Autodesk Inventor part; units mm, degrees
ref_plane "YZ Plane" through (0, 0, 0) normal (1, 0, 0) x (0, 1, 0)
ref_plane "XZ Plane" through (0, 0, 0) normal (0, 1, 0) x (-1, 0, 0)
ref_plane "XY Plane" through (0, 0, 0) normal (0, 0, 1) x (1, 0, 0)
sketch "Skizze1" plane through (0, 0, 0) normal (0, 1, 0) x (-1, 0, 0)
  line L0 (-27, 70) -> (27, 70)
  line L1 (27, 70) -> (27, -70)
  line L2 (27, -70) -> (-27, -70)
  line L3 (-27, -70) -> (-27, 70)
  line L4 (-27, 70) -> (27, -70) construction
  line L5 (27, 70) -> (-27, -70) construction
  point P0 (0, 0)
  dimension "d0" = 54
  dimension "d1" = 140
extrude "Extrusion1" add sketch "Skizze1" along normal blind 15
sketch "Skizze2" plane through (0, 15, 0) normal (0, 1, 0) x (1, 0, 0)
  line L0 (24, -63) -> (-24, -63)
  line L1 (-24, -63) -> (-24, 63)
  line L2 (-24, 63) -> (24, 63)
  line L3 (24, 63) -> (24, -63)
  line L4 (24, -63) -> (-24, 63) construction
  line L5 (-24, -63) -> (24, 63) construction
  line L6 (-27, -70) -> (27, -70)
  line L7 (27, -70) -> (27, 70)
  line L8 (27, 70) -> (-27, 70)
  line L9 (-27, 70) -> (-27, -70)
  point P0 (0, 0)
  dimension "d4" = 3
  dimension "d7" = 7
extrude "Extrusion2" cut sketch "Skizze2" against normal blind 12 contours L0 L1 L2 L3
sketch "Skizze4" plane through (-27, 0, 70) normal (0, 0, 1) x (1, 0, 0)
  line L0 (54, 0) -> (0, 0)
  line L1 (54, 0) -> (54, 15)
  line L2 (0, 15) -> (54, 15)
  line L3 (0, 0) -> (0, 15)
  point P0 (27, 3.5)
  dimension "d23" = 3.5
hole "Bohrung1" at (0, 3.5, 70) direction (0, 0, -1) diameter 2.459 depth 5 tip angle 118
pattern_linear "Rechteckige Anordnung1" count 5 spacing 11 along (-1, 0, 0) count 2 spacing 8 along (0, 1, 0) of "Bohrung1" first direction both ways yes
mirror "Spiegeln1" about plane through (0, 0, 0) normal (0, 0, 1) of "Extrusion2", "Bohrung1", "Rechteckige Anordnung1"
sketch "Skizze6" plane through (0, 0, 0) normal (0, -1, 0) x (1, 0, 0)
  line L0 (-18, 18) -> (18, 18)
  line L1 (18, 18) -> (18, -18)
  line L2 (18, -18) -> (-18, -18)
  line L3 (-18, -18) -> (-18, 18)
  line L4 (-18, 18) -> (18, -18) construction
  line L5 (18, 18) -> (-18, -18) construction
  line L6 (0, 18) -> (0, -18) construction
  line L7 (-18, 0) -> (18, 0) construction
  point P0 (0, 0)
  dimension "d47" = 36
  dimension "d48" = 36
hole "Bohrung2" at (18, 0, 18) at (18, 0, 0) at (18, 0, -18) at (0, 0, -18) at (-18, 0, -18) at (-18, 0, 0) at (-18, 0, 18) at (0, 0, 18) direction (0, 1, 0) diameter 2.459 depth 8.8 tip angle 118
fillet "Rundung2" radius 4 4 edges at (-24, 9, -63) (24, 9, -63) (24, 9, 63) (-24, 9, 63)
properties part number "dynamixel_pro_frame_part1" material "Aluminium 6061"
Build history of the part. All positions in model axes, mm. A direction names the side the tool comes from. Coordinates: 2 decimals unless noted, no trailing zeros. Order: outer loops, then holes, each group sorted by start corner. A loop starts at its lowest first (then second) coordinate and runs counter-clockwise, first axis right, second up. Notation, with made-up numbers: (62.5, 23.25) -> (81.5, 23.25) arc R11 ccw to (81.5, 36.25) -> close; hole circle Ø8 at (28.25, -31). An arc over 180 degrees is marked (long way). Answer in a Markdown table with one row per item. Add a question column.
Q1. Mould opens along Z. For faces 6 (the face through (-22.797, 8.916, 61.859)), 7 (the face through (10.631, 10.327, 67.465)), 8 (the face through (11.18, 11.39, 64.39)) say: +Z half, -Z half, draft (parallel to the pull), parting line (faces both ways), or undercut.
Q2. Wall check: line 1 along X through (y, z) = (11.5, 67.2); line 2 along Y through (x, z) = (11, -66.4); line 3 along X through (y, z) = (1.65, 18). Give the ranges that are in metal, low to high. Write a range as [from, to].
Q3. Band-saw the part on B-B, the plane z = 32. List the corners of the cut face in (x, y).
Q4. Band-saw the part on C-C, the plane x = 2.5. List the corners of the cut face in (y, z).
Q5. Which spindle directions (+Z, -Z, +X, -X, +Y, -Y) get a long thin tool onto all of the face, cutting with end or side? Do faces 1 (the face through (0.05, 4.73, -67.46)), 2 (the face through (-27, 7, 1)), 3 (the face through (0, 9, 63)), 4 (the face through (23.2, 3.77, 67.46)), 5 (the face through (0.471, 1.521, -19.136)). Say none if no direction does.
Q6. Band-saw the part on A-A, the plane z = -18. List the corners of the cut face in (x, y), then the cut area to 3 significant figures.
Q7. Drop flat-ended pins along their axis: pin 1 (1.5 mm diameter, centred on x = 11, y = 11.5, fed in from -Z); pin 2 (1.5 mm diameter, centred on x = 11, y = 3.5, fed in from +Z); pin 3 (1.5 mm diameter, centred on x = 17.5, z = 16, fed in from +Y); pin 4 (2 mm diameter, centred on x = 0, z = -18, fed in from +Y). Give the stop position or say it passes through.
Answers follow:
| question | item | result |
|---|---|---|
| 1 | face 6 | undercut |
| 1 | face 7 | draft |
| 1 | face 8 | +Z half |
| 2 | line 1 | [-27, -23.23], [-20.77, -12.23], [-9.77, -1.23], [1.23, 9.77], [12.23, 20.77], [23.23, 27] |
| 2 | line 2 | [0, 2.27], [4.73, 10.27], [12.73, 15] |
| 2 | line 3 | [-27, -19.23], [-16.77, -1.23], [1.23, 16.77], [19.23, 27] |
| 3 | outline | (-27, 0) -> (27, 0) -> (27, 15) -> (24, 15) -> (24, 3) -> (-24, 3) -> (-24, 15) -> (-27, 15) -> close |
| 4 | outline | (0, -70) -> (15, -70) -> (15, -63) -> (3, -63) -> (3, 63) -> (15, 63) -> (15, 70) -> (0, 70) -> close |
| 5 | face 1 | -Z |
| 5 | face 2 | +Z, -Z, -X, +Y, -Y |
| 5 | face 3 | +Y |
| 5 | face 4 | +Z |
| 5 | face 5 | +Y, -Y |
| 6 | outline | (-27, 0) -> (-19.23, 0) -> (-19.23, 3) -> (-24, 3) -> (-24, 15) -> (-27, 15) -> close; (-16.77, 0) -> (-1.23, 0) -> (-1.23, 3) -> (-16.77, 3) -> close; (1.23, 0) -> (16.77, 0) -> (16.77, 3) -> (1.23, 3) -> close; (19.23, 0) -> (27, 0) -> (27, 15) -> (24, 15) -> (24, 3) -> (19.23, 3) -> close |
| 6 | area | 212 mm^2 |
| 7 | pin 1 | z = -64.71 |
| 7 | pin 2 | z = 64.71 |
| 7 | pin 3 | y = 3 |
| 7 | pin 4 | through |
